CAD build for the part. Positions are in the model's coordinates, mm. Face numbers are marked on the shaded views. A direction names the side the tool comes from. Round coordinates to 2 decimals unless told otherwise and drop trailing zeros. Loops run counter-clockwise (first coordinate to the right, second up) from the corner with the lowest first, then second, coordinate; pieces in that order, holes last. Notation, with made-up numbers: M 13,-4 L 66,-4 A16 ccw 66,5 Z; hole C 64.5,-16 d8. An arc over 180 degrees is marked long. Use a Markdown table: item, result. Add a question column.
(1) Flat gauge pins, fed straight in: P1, Ø10, axis at y = -1.5, z = 8, coming from the -X side; P2, Ø2, axis at y = -12, z = 6, coming from the +X side; P3, Ø2, axis at x = 9.5, y = 9, coming from the +Z side; P4, Ø7, axis at x = 12, y = -20.5, coming from the +Z side. Where does each tip first touch, or does it go through?
(2) Band-saw the part on B-B, the plane z = 9.25. Write the cut outline in (x, y).
(3) Two-plate mould, pull along Y, no slides. Class the marked faces 1, 2, 3 and 4: released by +Y, released by -Y, zero draft, split by the parting line, or undercut.
(4) Wall check: L1, parallel to Y at x = 11, z = 8.25; L2, parallel to Z at x = 1.4, y = 20; L3, parallel to Y at x = 1.7, z = 10. Give the ranges that are in metal, low to high.
(5) Band-saw the part on C-C, the plane x = 4. Write the cut outline in (y, z), and give its area (3 significant figures).
(6) Band-saw the part on D-D, the plane z = 6.5. Write the cut outline in (x, y).
(7) Band-saw the part on A-A, the plane y = 20. Write the cut outline in (x, z).
(8) Which spindle directions (+Z, -Z, +X, -X, +Y, -Y) get a long thin tool onto all of the face, cutting with end or side? Do the marked faces 5 and 6. Say none if no direction does.
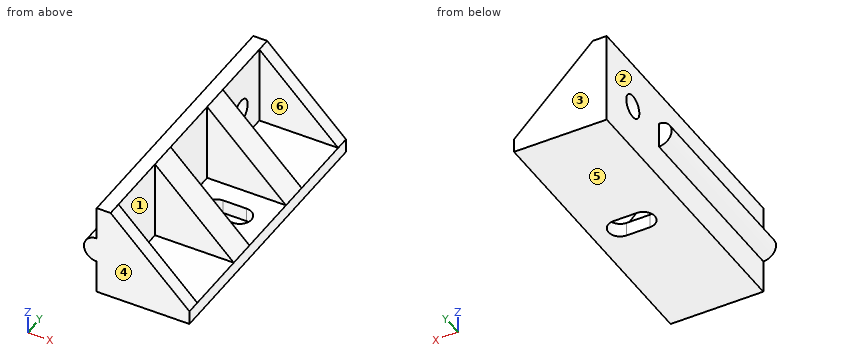
from build123d import *

# Parameters (mm, degrees)
BOX_W            = 20
BOX_H            = 20
BOX_DEPTH        = 20
EXTRUDE001_DEPTH = 50
CYLINDER_R       = 2.5
CYLINDER_DEPTH   = 10
BOX001_W         = 20
BOX001_H         = 14
BOX001_DEPTH     = 20
ARRAY_Y_COUNT    = 3
ARRAY_Y_PITCH    = 20
EXTRUDE_DEPTH    = 30


with BuildPart() as bolt_item_cube_cutter:
    # Box → Box (new body)
    with BuildSketch(Plane(origin=(-20, 10, 0), x_dir=(1, 0, 0), z_dir=(0, 0, 1))):
        with Locations((10, 10)):
            Rectangle(BOX_W, BOX_H)
    extrude(amount=BOX_DEPTH)


with BuildPart() as bottom_bolt_hole_extrude:
    # Sketch001 → Extrude001 (new body)
    with BuildSketch(Plane.XY):
        with BuildLine():
            ThreePointArc((-2.5, 2.5), (-5, 0), (-2.5, -2.5))
            Line((-2.5, -2.5), (2.5, -2.5))
            ThreePointArc((2.5, -2.5), (5, 0), (2.5, 2.5))
            Line((2.5, 2.5), (-2.5, 2.5))
        make_face()
    extrude(amount=EXTRUDE001_DEPTH)


with BuildPart() as bottom_bolt_hole_extrude_1:
    # Extrude001 placement: moved
    add(bottom_bolt_hole_extrude.part.moved(Location((11.5, 0, 0))))


with BuildPart() as bolt_hole:
    # Cylinder → Cylinder (new body)
    with BuildSketch(Plane(origin=(-5, 20, 10), x_dir=(0, 0, -1), z_dir=(1, 0, 0))):
        Circle(CYLINDER_R)
    extrude(amount=CYLINDER_DEPTH)


with BuildPart() as leg_extract:
    # Box001 → Box001 (new body)
    with BuildSketch(Plane(origin=(3, -27, 3), x_dir=(1, 0, 0), z_dir=(0, 0, 1))):
        with Locations((10, 7)):
            Rectangle(BOX001_W, BOX001_H)
    extrude(amount=BOX001_DEPTH)

    # Array Y: leg extract ×3


with BuildPart() as leg_extract_1:
    add(leg_extract.part)
    with Locations(*[(0, i * ARRAY_Y_PITCH, 0) for i in range(1, ARRAY_Y_COUNT)]):
        add(leg_extract.part)

    # Fusion: union bolt item cube cutter, bottom bolt hole extrude, bolt hole
    add(bolt_item_cube_cutter.part)
    add(bottom_bolt_hole_extrude_1.part)
    add(bolt_hole.part)


with BuildPart() as leg_cut:
    # Sketch → Extrude (new body, symmetric)
    with BuildSketch(Plane.XZ):
        with BuildLine():
            Line((0, 20), (3, 20))
            Line((3, 20), (20, 3))
            Line((20, 3), (20, 0))
            Line((20, 0), (0, 0))
            Line((0, 0), (0, 7.25))
            ThreePointArc((0, 12.75), (-2.75, 10), (0, 7.25))
            Line((0, 20), (0, 12.75))
        make_face()
    extrude(amount=EXTRUDE_DEPTH, both=True)

    # Cut: cut leg extract
    add(leg_extract_1.part, mode=Mode.SUBTRACT)


solid = leg_cut.part
Return value:
| question | item | result |
|---|---|---|
| 1 | P1 | x = -2.75 |
| 1 | P2 | x = 18 |
| 1 | P3 | z = 14.5 |
| 1 | P4 | z = 3 |
| 2 | outline | M -2.65,-30 L 13.75,-30 L 13.75,-27 L 3,-27 L 3,-13 L 13.75,-13 L 13.75,-7 L 3,-7 L 3,7 L 13.75,7 L 13.75,13 L 3,13 L 3,17.62 L 0,17.62 L 0,10 L -2.65,10 Z; M 0,22.38 L 3,22.38 L 3,27 L 13.75,27 L 13.75,30 L 0,30 Z |
| 3 | face 1 | undercut |
| 3 | face 2 | zero draft |
| 3 | face 3 | released by +Y |
| 3 | face 4 | released by -Y |
| 4 | L1 | -30 to -27, -13 to -7, 7 to 13, 27 to 30 |
| 4 | L2 | 0 to 7.5, 12.5 to 20 |
| 4 | L3 | -30 to 17.5, 22.5 to 30 |
| 5 | outline | M -30,0 L 30,0 L 30,19 L 27,19 L 27,3 L 13,3 L 13,19 L 7,19 L 7,3 L -7,3 L -7,19 L -13,19 L -13,3 L -27,3 L -27,19 L -30,19 Z |
| 5 | area | 468 mm^2 |
| 6 | outline | M 0,-30 L 16.5,-30 L 16.5,-27 L 3,-27 L 3,-13 L 16.5,-13 L 16.5,-7 L 3,-7 L 3,7 L 16.5,7 L 16.5,13 L 3,13 L 3,27 L 16.5,27 L 16.5,30 L 0,30 Z |
| 7 | outline | M 0,0 L 20,0 L 20,3 L 3,3 L 3,7.5 L 0,7.5 Z; M 0,12.5 L 3,12.5 L 3,20 L 0,20 Z |
| 8 | face 5 | -Z, +X, -X, +Y, -Y |
| 8 | face 6 | +Z, +X |
